from build123d import *

# Parameters (mm, degrees)
BOSS_EXTRUDE1_DEPTH = 10
SKETCH2_R           = 7.5
CUT_EXTRUDE1_DEPTH  = 13.5


with BuildPart() as part:
    # Sketch1 → Boss-Extrude1 (new body)
    with BuildSketch(Plane.XY):
        Polygon((0, -7.5), (6.495190528, -3.75), (6.495190528, 3.75), (0, 7.5), (-6.495190528, 3.75), (-6.495190528, -3.75), align=None)
    extrude(amount=BOSS_EXTRUDE1_DEPTH)

    # Sketch2 → Cut-Extrude1 (cut, symmetric)
    with BuildSketch(Plane(origin=(0, 0, 0), x_dir=(0, 0, -1), z_dir=(0, 1, 0))):
        with Locations((-13.75, 0)):
            Circle(SKETCH2_R)
    extrude(amount=CUT_EXTRUDE1_DEPTH, both=True, mode=Mode.SUBTRACT)


solid = part.part
The model under review builds one solid part; all positions refer to its coordinate system, in mm. Coordinates: 2 decimals unless noted, no trailing zeros. Write each loop counter-clockwise with the first axis right and the second up, starting at its lowest first coordinate (ties: lowest second). Pieces come first, ordered by that corner, then holes. Notation, with made-up numbers: (-1.5, -15) - (10.5, -15) arc R11 ccw to (10.5, -5) - close; hole circle Ø10 at (16.5, 63.25). An arc over 180 degrees is marked (long way). Answer as a JSON object with one key per item and string values. Group by question number.
1. Add section C-C (y = -2.75). Give the boundary of the cut face in (x, z).
2. Add section D-D (x = 2.5). Give the boundary of the cut face in (y, z).
3. Add section A-A (z = 8.25). Give the boundary of the cut face in (x, y), plus the area to 3 significant figures.
4. To check wall thickness, follow probe 1 along X at (y, z) = (2, 9); probe 2 along Z at (x, y) = (-0.25, -2.5); probe 3 along Z at (x, y) = (1.25, -2). State the ranges of each line that lie inside material, in increasing order.
5. Mouldability with a two-part tool opening along X and no side actions: class faces 1 (the face through (0, 0, 0)), 2 (the face through (-6.495, 0, 5)), 3 (the face through (0.11, 0.1, 6.25)), 4 (the face through (3.202, -5.651, 3.819)) as pulls with the +X half, pulls with the -X half, needs draft (parallel to the pull), parting line crosses it, or undercut.
6. Add section B-B (z = 3.75). Give the boundary of the cut face in (x, y), plus the area to 3 significant figures.
7. Clearance check with flat-ended pins moving along their axes: pin 1 Ø2 at (x, y) = (0, -2.5) entering from +Z; pin 2 Ø1.5 at (x, y) = (-1, 0.5) entering from -Z. State where each tip first meets the part, or that it passes through.
Findings:
{
 "1": {"outline": "(-6.5, 0) - (6.5, 0) - (6.5, 10) arc R7.5 cw to (-6.5, 10) - close"},
 "2": {"outline": "(-6.06, 0) - (6.06, 0) - (6.06, 6.68) - (-6.06, 6.68) - close"},
 "3": {"outline": "(-6.5, -3.75) - (-5.1, -4.56) - (-5.1, 4.56) - (-6.5, 3.75) - close; (5.1, -4.56) - (6.5, -3.75) - (6.5, 3.75) - (5.1, 4.56) - close", "area": "23.2 mm²"},
 "4": {"probe 1": "-6.5 to -5.8, 5.8 to 6.5", "probe 2": "0 to 6.25", "probe 3": "0 to 6.35"},
 "5": {"face 1": "needs draft", "face 2": "pulls with the -X half", "face 3": "undercut", "face 4": "pulls with the +X half"},
 "6": {"outline": "(-6.5, -3.75) - (0, -7.5) - (6.5, -3.75) - (6.5, 3.75) - (0, 7.5) - (-6.5, 3.75) - close", "area": "146 mm²"},
 "7": {"pin 1": "z = 6.32", "pin 2": "z = 0"}
}
